Drawing for the job (mm, zero at the part's lowest x, y, z). A direction names the side the tool comes from. Round coordinates to 2 decimals unless told otherwise and drop trailing zeros. Write each loop counter-clockwise with the first axis right and the second up, starting at its lowest first coordinate (ties: lowest second). Pieces come first, ordered by that corner, then holes. Notation, with made-up numbers: (-9.5, 57) - (25.5, 57) arc R21 cw to (25.5, 69) - close; hole circle Ø6 at (-37, 22.5). An arc over 180 degrees is marked (long way). One line per question, with ' | ' between items.
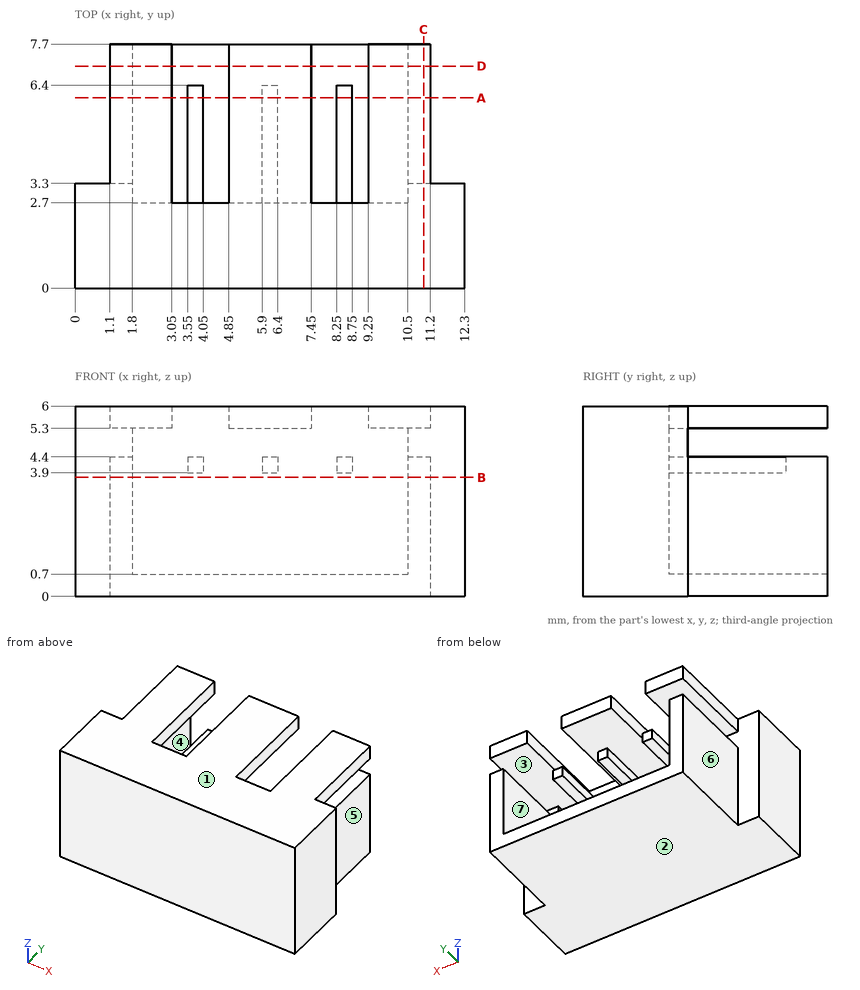
Q1. Pull direction Z, two halves, no side cores. Call the marked faces 1, 2, 3 and 4: +Z half, -Z half, draft (parallel to the pull), parting line (faces both ways), or undercut.
Found:
face 1: +Z half | face 2: -Z half | face 3: undercut | face 4: undercut
Q2. Saw through at B-B, the plane z = 3.75. List the corners of the cut face in (x, y), then the cut area to 3 significant figures.
Found:
outline: (0, 0) - (12.3, 0) - (12.3, 3.3) - (11.2, 3.3) - (11.2, 7.7) - (10.5, 7.7) - (10.5, 2.7) - (1.8, 2.7) - (1.8, 7.7) - (1.1, 7.7) - (1.1, 3.3) - (0, 3.3) - close | area: 41.5 mm^2
Q3. Saw through at C-C, the plane x = 11. List the corners of the cut face in (y, z).
Found:
outline: (0, 0) - (7.7, 0) - (7.7, 4.4) - (3.3, 4.4) - (3.3, 5.3) - (7.7, 5.3) - (7.7, 6) - (0, 6) - close
Q4. Saw through at D-D, the plane y = 7. List the corners of the cut face in (x, z).
Found:
outline: (1.1, 0) - (11.2, 0) - (11.2, 4.4) - (10.5, 4.4) - (10.5, 0.7) - (1.8, 0.7) - (1.8, 4.4) - (1.1, 4.4) - close; (1.1, 5.3) - (3.05, 5.3) - (3.05, 6) - (1.1, 6) - close; (4.85, 5.3) - (7.45, 5.3) - (7.45, 6) - (4.85, 6) - close; (9.25, 5.3) - (11.2, 5.3) - (11.2, 6) - (9.25, 6) - close
Q5. Drill centre lines: L1, parallel to X at y = 6.5, z = 5.65; L2, parallel to X at y = 3.25, z = 4; L3, parallel to Z at x = 10, y = 5.5. Where is each one in solid material? Low to high. Write a range as from..to.
Found:
L1: 1.1..3.05, 4.85..7.45, 9.25..11.2 | L2: 0..1.8, 3.55..4.05, 5.9..6.4, 8.25..8.75, 10.5..12.3 | L3: 0..0.7, 5.3..6
Q6. Saw through at A-A, the plane y = 6. State how many separate pieces and enclosed holes the cut face has, then the cut area to 4 significant figures.
Found:
separate pieces: 7 | enclosed holes: 0 | area: 17.55 mm^2
Q7. Drop flat-ended pins along their axis: pin 1 (2.5 mm diameter, centred on y = 5.5, z = 3, fed in from +X); pin 2 (1 mm diameter, centred on x = 6, z = 1.5, fed in from +Y); pin 3 (0.6 mm diameter, centred on y = 4.5, z = 5.5, fed in from -X). Give the stop position or say it passes through.
Found:
pin 1: x = 11.2 | pin 2: y = 2.7 | pin 3: x = 1.1
Q8. Which spindle directions (+Z, -Z, +X, -X, +Y, -Y) get a long thin tool onto all of the face, cutting with end or side? Do the marked faces 5, 6 and 7. Say none if no direction does.
Found:
face 5: +Z, -Z, +X, +Y | face 6: +Z, -Z, -X, +Y | face 7: +Y
